Can you work these out from the model? Positions are in its coordinate system, mm. Face numbers are marked on the shaded views. A direction names the side the tool comes from. Round coordinates to 2 decimals unless told otherwise and drop trailing zeros. Order: outer loops, then holes, each group sorted by start corner. A loop starts at its lowest first (then second) coordinate and runs counter-clockwise, first axis right, second up. Notation, with made-up numbers: (-30.5, 46.5) - (26.5, 46.5) arc R17 cw to (26.5, 75.5) - close; hole circle Ø10 at (-31.75, 66.25). An arc over 180 degrees is marked (long way). Write item = value, one per line.
from build123d import *

# Parameters (mm, degrees)
SKETCH1_W           = 100
SKETCH1_H           = 20
SKETCH1_R           = 6.1
SKETCH1_R_2         = 4.1
BOSS_EXTRUDE1_DEPTH = 40
SKETCH2_W           = 100
SKETCH2_H           = 20
BOSS_EXTRUDE2_DEPTH = 33.4
CUT_EXTRUDE1_REACH  = 111.545
SKETCH3_W           = 58.5
SKETCH3_H           = 49


with BuildPart() as part:
    # Sketch1 → Boss-Extrude1 (new body)
    with BuildSketch(Plane.XY):
        with Locations((-50, 10)):
            Rectangle(SKETCH1_W, SKETCH1_H)
        with Locations((-90, 10)):
            Circle(SKETCH1_R, mode=Mode.SUBTRACT)
        with Locations((-66.5, 10)):
            Circle(SKETCH1_R_2, mode=Mode.SUBTRACT)
    boss_extrude1 = extrude(amount=BOSS_EXTRUDE1_DEPTH)

    # Sketch2 → Boss-Extrude2 (add)
    with BuildSketch(Plane(origin=(0, 0, 0), x_dir=(-1, 0, 0), z_dir=(0, 0, -1))):
        with Locations((50, 10)):
            Rectangle(SKETCH2_W, SKETCH2_H)
    boss_extrude2 = extrude(amount=BOSS_EXTRUDE2_DEPTH)

    # Sketch3 → Cut-Extrude1 (cut, up to next)
    with BuildSketch(Plane(origin=(0, 20, 0), x_dir=(1, 0, 0), z_dir=(0, 1, 0)), mode=Mode.PRIVATE) as cut_extrude1_sk1:
        with Locations((-29.25, -3.3)):
            Rectangle(SKETCH3_W, SKETCH3_H)
    cut_extrude1_tool1 = extrude(cut_extrude1_sk1.sketch, amount=-CUT_EXTRUDE1_REACH, mode=Mode.PRIVATE) & part.part
    cut_extrude1 = cut_extrude1_tool1.solids().sort_by_distance((-29.25, 20, 3.3))[0]
    add(cut_extrude1, mode=Mode.SUBTRACT)

    # Mirror2: Boss-Extrude1, Boss-Extrude2, Cut-Extrude1 across plane
    add(boss_extrude1.mirror(Plane(origin=(0, 0, 40), x_dir=(0, 0, 1), z_dir=(-1, 0, 0))))
    add(boss_extrude2.mirror(Plane(origin=(0, 0, 40), x_dir=(0, 0, 1), z_dir=(-1, 0, 0))))
    add(cut_extrude1.mirror(Plane(origin=(0, 0, 40), x_dir=(0, 0, 1), z_dir=(-1, 0, 0))), mode=Mode.SUBTRACT)


solid = part.part
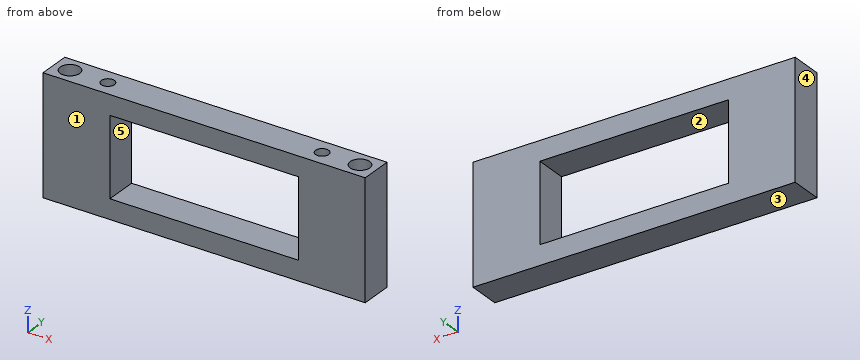
(1) If we section it at B-B (x = -30): Write out the boundary of the cut face in (y, z), plus the area to 3 significant figures.
Computed:
outline = (0, -33.4) - (20, -33.4) - (20, -21.2) - (0, -21.2) - close; (0, 27.8) - (20, 27.8) - (20, 40) - (0, 40) - close
area = 488 mm^2
(2) If we section it at C-C (y = 18): Write out the boundary of the cut face in (x, z).
Computed:
outline = (-100, -33.4) - (100, -33.4) - (100, 40) - (-100, 40) - close; hole (-58.5, -21.2) - (58.5, -21.2) - (58.5, 27.8) - (-58.5, 27.8) - close
(3) On a 3-axis mill with a long thin cutter (end or side, diameter ignored), from which of +Z, -Z, +X, -X, +Y, -Y can I reach the whole of each face in a straight line? I mean the marked faces 4 and 5. Say none if no direction works.
Computed:
face_4 = +Z, -Z, -X, +Y, -Y
face_5 = +Y, -Y
(4) Thinking about a two-plate mould opening in Z: for the marked faces 1, 2 and 3, which applies, +Z half, -Z half, draft (parallel to the pull), parting line (faces both ways), or undercut?
Computed:
face_1 = draft
face_2 = undercut
face_3 = -Z half
(5) If I drill on line 1 (Z direction, x = -5.5, y = 8); line 2 (X direction, y = 1.5, z = 15); line 3 (Y direction, x = 90, z = 27), over which ranges is the centre line in solid material (lowest first)? Write a range as from..to.
Computed:
line_1 = -33.4..-21.2, 27.8..40
line_2 = -100..-58.5, 58.5..100
line_3 = 0..3.9, 16.1..20
(6) Will this pin go through, and if not, where does the flat tip stop? P1, Ø6.5, axis at x = -66.5, y = 10, coming from the +Z side.
Computed:
P1 = 0
(7) If we section it at D-D (x = -66.5): Write out the boundary of the cut face in (y, z), plus the area to 3 significant figures.
Computed:
outline = (0, -33.4) - (20, -33.4) - (20, 40) - (14.1, 40) - (14.1, 0) - (5.9, 0) - (5.9, 40) - (0, 40) - close
area = 1,140 mm^2
(8) If we section it at A-A (z = 4.5): Write out the boundary of the cut face in (x, y), plus the area to 3 significant figures.
Computed:
outline = (-100, 0) - (-58.5, 0) - (-58.5, 20) - (-100, 20) - close; (58.5, 0) - (100, 0) - (100, 20) - (58.5, 20) - close; hole circle Ø12.2 at (-90, 10); hole circle Ø8.2 at (-66.5, 10); hole circle Ø8.2 at (66.5, 10); hole circle Ø12.2 at (90, 10)
area = 1,320 mm^2
